```python
from build123d import *

# Parameters (mm, degrees)
SKETCH2_W           = 66.5
SKETCH2_H           = 63.5
BOSS_EXTRUDE1_DEPTH = 3
SKETCH3_W           = 62.5
SKETCH3_H           = 60.25
CUT_EXTRUDE1_DEPTH  = 0.75
SKETCH4_W           = 42
SKETCH4_H           = 56.75
CUT_EXTRUDE2_DEPTH  = 47.029202687
SKETCH6_W           = 72
SKETCH6_H           = 69
SKETCH6_W_2         = 66.5
SKETCH6_H_2         = 63.5
BOSS_EXTRUDE2_DEPTH = 33
SKETCH7_W           = 60.5
SKETCH7_H           = 30
CUT_EXTRUDE3_DEPTH  = 30
SKETCH8_W           = 11
SKETCH8_H           = 10
CUT_EXTRUDE4_DEPTH  = 3
SKETCH10_W          = 32
SKETCH10_H          = 16.5
CUT_EXTRUDE5_DEPTH  = 16.5
BOSS_EXTRUDE3_DEPTH = 1.3
SKETCH12_W          = 15
SKETCH12_H          = 3
CUT_EXTRUDE6_DEPTH  = 86.049926514
SKETCH13_W          = 15
SKETCH13_H          = 3
CUT_EXTRUDE7_DEPTH  = 3
SKETCH14_W          = 16.4
SKETCH14_H          = 4.4
SKETCH14_W_2        = 15
SKETCH14_H_2        = 3
CUT_EXTRUDE9_DEPTH  = 1.55
SKETCH15_W          = 15
SKETCH15_H          = 1.75
CUT_EXTRUDE10_DEPTH = 4
SKETCH17_W          = 16.4
SKETCH17_H          = 4.4
SKETCH17_W_2        = 15
SKETCH17_H_2        = 3
CUT_EXTRUDE12_DEPTH = 1.5
SKETCH16_W          = 1.75
SKETCH16_H          = 15
CUT_EXTRUDE11_DEPTH = 4
SKETCH18_W          = 28
SKETCH18_H          = 3
CUT_EXTRUDE13_DEPTH = 3
SKETCH20_W          = 2.75
SKETCH20_H          = 60.5
BOSS_EXTRUDE4_DEPTH = 2.7


with BuildPart() as part:
    # Sketch2 → Boss-Extrude1 (new body)
    with BuildSketch(Plane(origin=(0, 0, 0), x_dir=(1, 0, 0), z_dir=(0, 1, 0))):
        Rectangle(SKETCH2_W, SKETCH2_H)
    extrude(amount=BOSS_EXTRUDE1_DEPTH)

    # Sketch3 → Cut-Extrude1 (cut)
    with BuildSketch(Plane(origin=(0, 3, 0), x_dir=(1, 0, 0), z_dir=(0, 1, 0))):
        with Locations((-2, 0)):
            Rectangle(SKETCH3_W, SKETCH3_H)
    extrude(amount=-CUT_EXTRUDE1_DEPTH, mode=Mode.SUBTRACT)

    # Sketch4 → Cut-Extrude2 (cut, through all)
    with BuildSketch(Plane(origin=(0, 2.25, 0), x_dir=(1, 0, 0), z_dir=(0, 1, 0))):
        with Locations((6.25, 0.25)):
            Rectangle(SKETCH4_W, SKETCH4_H)
    extrude(amount=-CUT_EXTRUDE2_DEPTH, mode=Mode.SUBTRACT)

    # Sketch6 → Boss-Extrude2 (add)
    with BuildSketch(Plane(origin=(0, 0, 0), x_dir=(1, 0, 0), z_dir=(0, 1, 0))):
        Rectangle(SKETCH6_W, SKETCH6_H)
        Rectangle(SKETCH6_W_2, SKETCH6_H_2, mode=Mode.SUBTRACT)
    extrude(amount=BOSS_EXTRUDE2_DEPTH)

    # Sketch7 → Cut-Extrude3 (cut)
    with BuildSketch(Plane.ZY.offset(36)):
        with Locations((-0.25, 18)):
            Rectangle(SKETCH7_W, SKETCH7_H)
    extrude(amount=-CUT_EXTRUDE3_DEPTH, mode=Mode.SUBTRACT)

    # Sketch8 → Cut-Extrude4 (cut)
    with BuildSketch(Plane(origin=(36, 0, 0), x_dir=(0, 0, -1), z_dir=(1, 0, 0))):
        with Locations((-20, 8.5)):
            Rectangle(SKETCH8_W, SKETCH8_H)
    extrude(amount=-CUT_EXTRUDE4_DEPTH, mode=Mode.SUBTRACT)

    # Sketch10 → Cut-Extrude5 (cut)
    with BuildSketch(Plane(origin=(0, 0, -34.5), x_dir=(-1, 0, 0), z_dir=(0, 0, -1))):
        with Locations((-7, 24.75)):
            Rectangle(SKETCH10_W, SKETCH10_H)
    extrude(amount=-CUT_EXTRUDE5_DEPTH, mode=Mode.SUBTRACT)

    # Sketch11 → Boss-Extrude3 (add)
    with BuildSketch(Plane(origin=(0, 33, 0), x_dir=(1, 0, 0), z_dir=(0, 1, 0))):
        with BuildLine():
            Line((-34.25, 31.25), (-34.25, 30.5))
            Line((-34.25, 30.5), (-33.25, 30.5))
            Line((-33.25, 30.5), (-33.25, 31.75))
            Line((-33.25, 31.75), (-9, 31.75))
            Line((-9, 31.75), (-9, 32.75))
            Line((-9, 32.75), (-32.75, 32.75))
            ThreePointArc((-32.75, 32.75), (-33.810660172, 32.310660172), (-34.25, 31.25))
        make_face()
        with BuildLine():
            Line((-33.25, -31.75), (33.25, -31.75))
            Line((33.25, -31.75), (33.25, 31.75))
            Line((33.25, 31.75), (23, 31.75))
            Line((23, 31.75), (23, 32.75))
            Line((23, 32.75), (32.75, 32.75))
            ThreePointArc((32.75, 32.75), (33.810660172, 32.310660172), (34.25, 31.25))
            Line((34.25, 31.25), (34.25, -31.25))
            ThreePointArc((34.25, -31.25), (33.810660172, -32.310660172), (32.75, -32.75))
            Line((32.75, -32.75), (-32.75, -32.75))
            ThreePointArc((-32.75, -32.75), (-33.810660172, -32.310660172), (-34.25, -31.25))
            Line((-34.25, -31.25), (-34.25, -30))
            Line((-34.25, -30), (-33.25, -30))
            Line((-33.25, -30), (-33.25, -31.75))
        make_face()
    extrude(amount=BOSS_EXTRUDE3_DEPTH)

    # Sketch12 → Cut-Extrude6 (cut, through all)
    with BuildSketch(Plane.XY.offset(34.5)):
        with Locations((-18.5, 30.5)):
            Rectangle(SKETCH12_W, SKETCH12_H)
    extrude(amount=-CUT_EXTRUDE6_DEPTH, mode=Mode.SUBTRACT)

    # Sketch13 → Cut-Extrude7 (cut)
    with BuildSketch(Plane(origin=(36, 0, 0), x_dir=(0, 0, -1), z_dir=(1, 0, 0))):
        with Locations((0, 30.5)):
            Rectangle(SKETCH13_W, SKETCH13_H)
    extrude(amount=-CUT_EXTRUDE7_DEPTH, mode=Mode.SUBTRACT)

    # Sketch14 → Cut-Extrude9 (cut)
    with BuildSketch(Plane.XY.offset(34.5)):
        with Locations((-18.5, 30.5)):
            Rectangle(SKETCH14_W, SKETCH14_H)
        with Locations((-18.5, 30.5)):
            Rectangle(SKETCH14_W_2, SKETCH14_H_2, mode=Mode.SUBTRACT)
    cut_extrude9 = extrude(amount=-CUT_EXTRUDE9_DEPTH, mode=Mode.SUBTRACT)

    # Sketch15 → Cut-Extrude10 (cut)
    with BuildSketch(Plane(origin=(0, 33, 0), x_dir=(1, 0, 0), z_dir=(0, 1, 0))):
        with Locations((-18.5, -33.625)):
            Rectangle(SKETCH15_W, SKETCH15_H)
    cut_extrude10 = extrude(amount=-CUT_EXTRUDE10_DEPTH, mode=Mode.SUBTRACT)

    # Mirror1: Cut-Extrude9, Cut-Extrude10 across plane
    add(cut_extrude9.mirror(Plane.XY), mode=Mode.SUBTRACT)
    add(cut_extrude10.mirror(Plane.XY), mode=Mode.SUBTRACT)

    # Sketch17 → Cut-Extrude12 (cut)
    with BuildSketch(Plane(origin=(36, 0, 0), x_dir=(0, 0, -1), z_dir=(1, 0, 0))):
        with Locations((0, 30.5)):
            Rectangle(SKETCH17_W, SKETCH17_H)
        with Locations((0, 30.5)):
            Rectangle(SKETCH17_W_2, SKETCH17_H_2, mode=Mode.SUBTRACT)
    extrude(amount=-CUT_EXTRUDE12_DEPTH, mode=Mode.SUBTRACT)

    # Sketch16 → Cut-Extrude11 (cut)
    with BuildSketch(Plane(origin=(0, 33, 0), x_dir=(1, 0, 0), z_dir=(0, 1, 0))):
        with Locations((35.125, 0.25)):
            Rectangle(SKETCH16_W, SKETCH16_H)
    extrude(amount=-CUT_EXTRUDE11_DEPTH, mode=Mode.SUBTRACT)

    # Sketch18 → Cut-Extrude13 (cut)
    with BuildSketch(Plane.XZ):
        with Locations((6.25, 29.625)):
            Rectangle(SKETCH18_W, SKETCH18_H)
    extrude(amount=-CUT_EXTRUDE13_DEPTH, mode=Mode.SUBTRACT)

    # Sketch20 → Boss-Extrude4 (add)
    with BuildSketch(Plane(origin=(0, 3, 0), x_dir=(1, 0, 0), z_dir=(0, 1, 0))):
        with Locations((-34.625, 0.25)):
            Rectangle(SKETCH20_W, SKETCH20_H)
    extrude(amount=BOSS_EXTRUDE4_DEPTH)


solid = part.part
```
Check sheet for the modelled part. Datum: model origin and axes. Units: mm. A direction names the side the tool comes from. Round coordinates to 2 decimals unless told otherwise and drop trailing zeros. Loops run counter-clockwise (first coordinate to the right, second up) from the corner with the lowest first, then second, coordinate; pieces in that order, holes last. Notation, with made-up numbers: (70, 52.25) - (104, 52.25) arc R32 cw to (104, 83.25) - close; hole circle Ø5 at (6.5, -18). An arc over 180 degrees is marked (long way). Answer as a JSON object with one key per item and string values. Group by question number.
Q1. Mould release check, pull along X, two halves, no side actions. Record for faces 5 (the face through (-35, 20, -30.5)), 6 (the face through (20.25, 1, 30)), 7 (the face through (0.5, 33.4, 32.75)): released by +X, released by -X, zero draft, split by the parting line, or undercut.
Q2. Sectioned sample at D-D, the plane z = 23. Enter the section's corners in (x, y).
Q3. Sectioned sample at B-B, the plane y = 18. Enter the section's corners in (x, z), plus the area to 3 significant figures.
Q4. Sectioned sample at C-C, the plane x = 19. Enter the section's corners in (y, z) (3 decimals).
Q5. Gauge pin test, flat ends, axial feed: P1, Ø22, axis at x = 16, z = 25, coming from the +Y side; P2, Ø0.9, axis at x = -10, z = -33.5, coming from the +Y side; P3, Ø2, axis at x = -21, y = 29.5, coming from the -Z side; P4, Ø1.5, axis at x = -29, z = -6, coming from the +Y side. Record the tip position at first contact, or that the pin passes through.
Q6. Scan lines: line 1 along Z through (x, y) = (26.5, 33.5); line 2 along Z through (x, y) = (-22, 9.5); line 3 along X through (y, z) = (19.5, -31). Record each from-to range of solid material in increasing order. Write a range as [from, to].
Q7. Set-up check for faces 1 (the face through (-33.25, 5, 7)), 2 (the face through (23, 25, -33)), 3 (the face through (35, 33, -24)), 4 (the face through (-7.75, 1, 30)): record each of +Z, -Z, +X, -X, +Y, -Y from which the full face is reachable in a straight line by a thin tool's end or side.
Q8. Sectioned sample at A-A, the plane z = -1. Enter the section's corners in (x, y), plus the area to 3 significant figures.
Solution:
{
 "1": {"face 5": "zero draft", "face 6": "undercut", "face 7": "undercut"},
 "2": {"outline": "(-36, 0) - (-14.75, 0) - (-14.75, 2.25) - (-33.25, 2.25) - (-33.25, 5.7) - (-36, 5.7) - close; (27.25, 0) - (36, 0) - (36, 3.5) - (33.25, 3.5) - (33.25, 3) - (29.25, 3) - (29.25, 2.25) - (27.25, 2.25) - close; (33.25, 13.5) - (36, 13.5) - (36, 33) - (34.25, 33) - (34.25, 34.3) - (33.25, 34.3) - close"},
 "3": {"outline": "(-36, -34.5) - (-9, -34.5) - (-9, -31.75) - (-33.25, -31.75) - (-33.25, -30.5) - (-36, -30.5) - close; (-36, 30) - (-33.25, 30) - (-33.25, 31.75) - (33.25, 31.75) - (33.25, -31.75) - (23, -31.75) - (23, -34.5) - (36, -34.5) - (36, 34.5) - (-36, 34.5) - close", "area": "491 mm²"},
 "4": {"outline": "(0, -34.5) - (16.5, -34.5) - (16.5, -31.75) - (3, -31.75) - (3, -30.125) - (2.25, -30.125) - (2.25, -28.625) - (0, -28.625) - close; (0, 31.125) - (3, 31.125) - (3, 31.75) - (34.3, 31.75) - (34.3, 32.75) - (33, 32.75) - (33, 34.5) - (0, 34.5) - close"},
 "5": {"P1": "stops at y = 34.3", "P2": "stops at y = 33", "P3": "stops at z = -32.95", "P4": "stops at y = 2.25"},
 "6": {"line 1": "z = [-32.75, -31.75], [31.75, 32.75]", "line 2": "z = [-34.5, -31.75], [31.75, 34.5]", "line 3": "x = [-36, -33.25], [33.25, 36]"},
 "7": {"face 1": "+Y", "face 2": "-Z, +Y", "face 3": "-Z, +X, +Y", "face 4": "+Y, -Y"},
 "8": {"outline": "(-36, 0) - (-14.75, 0) - (-14.75, 2.25) - (-33.25, 2.25) - (-33.25, 5.7) - (-36, 5.7) - close; (27.25, 0) - (36, 0) - (36, 28.3) - (34.5, 28.3) - (34.5, 29) - (33.25, 29) - (33.25, 3) - (29.25, 3) - (29.25, 2.25) - (27.25, 2.25) - close; (33.25, 32) - (34.25, 32) - (34.25, 34.3) - (33.25, 34.3) - close", "area": "155 mm²"}
}
